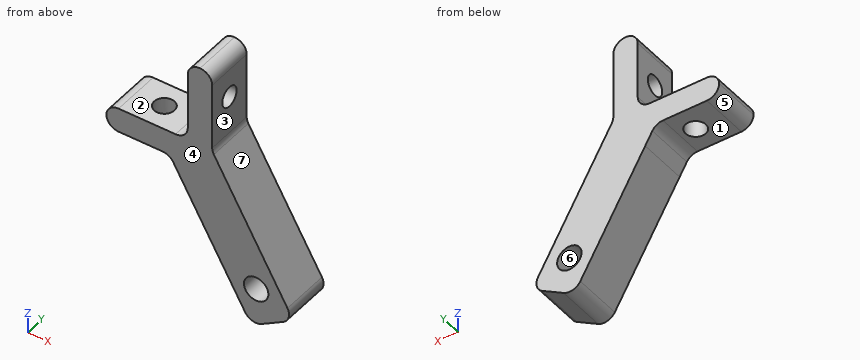
```python
from build123d import *

# Parameters (mm, degrees)
BOSS_EXTRUDE1_DEPTH      = 6
BOSS_EXTRUDE1_DEPTH_BACK = 6
SKETCH1_R                = 3
SKETCH2_R                = 2.5
CUT_EXTRUDE1_DEPTH       = 44.824009589
SKETCH3_R                = 2.5
CUT_EXTRUDE2_DEPTH       = 52.241882852
FILLET1_R                = 3


with BuildPart() as part:
    # Sketch1 → Boss-Extrude1 (new, two sides: drawn at the far end of the back side and taken through both)
    with BuildSketch(Plane(origin=(0, 0, 0), x_dir=(1, 0, 0), z_dir=(0, 1, 0)).offset(-BOSS_EXTRUDE1_DEPTH_BACK)):
        Polygon((0, 0), (-15.536622966, 0), (-15.536622966, -6), (4.463377034, -6), (4.463377034, -26), (10.463377034, -26), (10.463377034, -5.876899358), (30.463377034, 28.764116793), (20.071072189, 34.764116793), (2.632022894, 4.55879738), align=None)
        with Locations(Location((21.267224611, 24.835913563, 0), (0, 0, 270))):
            Circle(SKETCH1_R, mode=Mode.SUBTRACT)
    extrude(amount=BOSS_EXTRUDE1_DEPTH + BOSS_EXTRUDE1_DEPTH_BACK)

    # Sketch2 → Cut-Extrude1 (cut, through all)
    with BuildSketch(Plane.ZY.offset(-4.463377034)):
        with Locations((16, 0)):
            Circle(SKETCH2_R)
    extrude(amount=-CUT_EXTRUDE1_DEPTH, mode=Mode.SUBTRACT)

    # Sketch3 → Cut-Extrude2 (cut, through all)
    with BuildSketch(Plane.XY.offset(6)):
        with Locations((-5.536622966, 0)):
            Circle(SKETCH3_R)
    extrude(amount=-CUT_EXTRUDE2_DEPTH, mode=Mode.SUBTRACT)

    # Fillet1
    fillet1_edges = [part.edges().sort_by_distance(p)[0] for p in [
        (10.463377034, 0, 26),
        (4.463377034, 0, 26),
        (-15.536622966, 0, 6),
        (-15.536622966, 0, 0),
        (4.463377034, 0, 6),
        (10.463377034, 0, 5.876899358),
        (30.463377034, 0, -28.764116793),
        (20.071072189, 0, -34.764116793),
        (0, 0, 0),
    ]]
    fillet(fillet1_edges, radius=FILLET1_R - 0.0001)  # a hair under: the kernel refuses the full size


solid = part.part
```
The model under review builds one solid part; all positions refer to its coordinate system, in mm. Face numbers are marked on the shaded views. A direction names the side the tool comes from. Give positions to 0.01 mm unless a question says otherwise; leave off trailing zeros. Order: outer loops, then holes, each group sorted by start corner. A loop starts at its lowest first (then second) coordinate and runs counter-clockwise, first axis right, second up. Notation, with made-up numbers: (74.5, 86) - (125.5, 86) arc R20 ccw to (125.5, 92) - close; hole circle Ø8 at (17.5, -37). An arc over 180 degrees is marked (long way). Use CSV: the item, a comma, the result in double quotes. Start each with the question number.
Q1. We need section B-B, the plane y = -1.75. State how many separate pieces and enclosed holes the cut face has, and give its area (3 significant figures).
Q2. We need section C-C, the plane x = 22. Write out the cut boundary in (y, z), and give its area (3 significant figures).
Q3. The part is to be moulded in two halves that separate along Z. For the marked faces 4, 5, 6 and 7, say which applies: +Z half, -Z half, draft (parallel to the pull), parting line (faces both ways), or undercut.
Q4. Clearance check with flat-ended pins moving along their axes: pin 1 Ø1.5 at (y, z) = (-1, -1.5) entering from +X; pin 2 Ø5.5 at (x, y) = (-5.5, -1.5) entering from -Z; pin 3 Ø6 at (x, y) = (-7.5, 1) entering from +Z. State where each tip first meets the part, or that it passes through.
Q5. To check wall thickness, follow line 1 along Y through (x, z) = (6, 16); line 2 along X through (y, z) = (-1.75, -25); line 3 along X through (y, z) = (5, -24.5). State the ranges of each line that lie inside material, in increasing order. Write a range as [from, to].
Q6. We need section A-A, the plane z = 16. Write out the cut boundary in (x, y).
Q7. Tool access review of the marked faces 1, 2 and 3: name each direction out of +Z, -Z, +X, -X, +Y, -Y from which nothing blocks a thin tool from reaching the whole face with its end or side.
Outcome:
1,separate pieces,"3"
1,enclosed holes,"1"
1,area,"646 mm^2"
2,outline,"(-6, -33.55) - (6, -33.55) - (6, -27.75) - (-6, -27.75) - close; (-6, -21.93) - (6, -21.93) - (6, -14.11) - (-6, -14.11) - close"
2,area,"164 mm^2"
3,face 4,"draft"
3,face 5,"-Z half"
3,face 6,"undercut"
3,face 7,"+Z half"
4,pin 1,"stops at x = 15.16"
4,pin 2,"stops at z = 0"
4,pin 3,"stops at z = 6"
5,line 1,"y = [-6, -2.5], [2.5, 6]"
5,line 2,"x = [14.43, 18.27], [24.26, 28.29]"
5,line 3,"x = [14.15, 18.29], [24.25, 28]"
6,outline,"(4.46, -6) - (10.46, -6) - (10.46, -2.5) - (4.46, -2.5) - close; (4.46, 2.5) - (10.46, 2.5) - (10.46, 6) - (4.46, 6) - close"
7,face 1,"-Z, -X, +Y, -Y"
7,face 2,"+Z, -X, +Y, -Y"
7,face 3,"+Z, +X, +Y, -Y"
